CAD build for the part. Positions are in the model's coordinates, mm. A direction names the side the tool comes from. Round coordinates to 2 decimals unless told otherwise and drop trailing zeros. Order: outer loops, then holes, each group sorted by start corner. A loop starts at its lowest first (then second) coordinate and runs counter-clockwise, first axis right, second up. Notation, with made-up numbers: M -13.75,4.5 L 36.25,4.5 A9 cw 36.25,19.5 Z; hole C 50.25,29.25 d1. An arc over 180 degrees is marked long. Answer as a JSON object with one key per item and string values.
```python
from build123d import *

# Parameters (mm, degrees)
F0_W     = 127
F0_H     = 127
F1_DEPTH = 25.4
F2_R     = 5.08
F3_DEPTH = 25.4
F4_DEPTH = 25.4
F5_DEPTH = 25.399999693
F6_DEPTH = 25.4


with BuildPart() as f1:
    # F0 (on Top) → F1 (new body)
    with BuildSketch(Plane.XY):
        with Locations((-6.1427538668, 6.0419291258)):
            Rectangle(F0_W, F0_H)
    extrude(amount=F1_DEPTH)

    # F2
    f2_edges = [f1.edges().sort_by_distance(p)[0] for p in [
        (57.357246, -57.458071, 12.7),
        (57.357246, 69.541929, 12.7),
        (-69.642754, -57.458071, 12.7),
        (-69.642754, 69.541929, 12.7),
    ]]
    fillet(f2_edges, radius=F2_R)

    # F3 (add): a face of the model
    f3_faces = [f1.faces().sort_by_distance(p)[0] for p in [
        (-69.6427538668, 6.0419291258, 12.7),
    ]]
    extrude(f3_faces, amount=F3_DEPTH)

    # F4 (add): a face of the model
    f4_faces = [f1.faces().sort_by_distance(p)[0] for p in [
        (-95.0427538668, 6.0419291258, 12.7),
    ]]
    extrude(f4_faces, amount=F4_DEPTH)

    # F5 (add): a face of the model
    f5_faces = [f1.faces().sort_by_distance(p)[0] for p in [
        (-120.4427538668, 6.0419291258, 12.7),
    ]]
    extrude(f5_faces, amount=-F5_DEPTH)

    # F6 (add): a face of the model
    f6_faces = [f1.faces().sort_by_distance(p)[0] for p in [
        (-30.0814078041, 6.0419291258, 25.4),
    ]]
    extrude(f6_faces, amount=F6_DEPTH)


solid = f1.part
```
Item 1: Drop flat-ended pins along their axis: pin 1 Ø7.5 at (x, z) = (-104, 15.5) entering from +Y; pin 2 Ø2 at (x, z) = (-69.5, 45.5) entering from -Y. Give the stop position or say it passes through.
Worked answers:
{"pin 1": "stops at y = 64.46", "pin 2": "stops at y = -55.59"}
Item 2: Saw through at A-A on z = 5. List the corners of the cut face in (x, y).
Worked answers:
{"outline": "M -120.44,-52.38 L -69.64,-52.38 A5.08 ccw -64.56,-57.46 L 52.28,-57.46 A5.08 ccw 57.36,-52.38 L 57.36,64.46 A5.08 ccw 52.28,69.54 L -64.56,69.54 A5.08 ccw -69.64,64.46 L -120.44,64.46 Z"}
Item 3: Wall check: line 1 along Y through (x, z) = (-88, 3); line 2 along Y through (x, z) = (-68.5, 47). Give the ranges that are in metal, low to high. Write a range as [from, to].
Worked answers:
{"line 1": "y = [-52.38, 64.46]", "line 2": "y = [-55.59, 67.67]"}
Item 4: 3-axis set-ups, long thin cutter, end or side, ignore diameter. For faces 1 (the flat face through (-95, -52.378, 25)), 2 (the flat face through (-33, 5, 50.8)): which of +Z, -Z, +X, -X, +Y, -Y reach the whole face in a straight line?
Worked answers:
{"face 1": "+Z, -Z, -X, -Y", "face 2": "+Z, +X, -X, +Y, -Y"}
